Build history of the part. All positions in model axes, mm. Face numbers are marked on the shaded views. A direction names the side the tool comes from. Round coordinates to 2 decimals unless told otherwise and drop trailing zeros. Write each loop counter-clockwise with the first axis right and the second up, starting at its lowest first coordinate (ties: lowest second). Pieces come first, ordered by that corner, then holes.
from build123d import *

# Parameters (mm, degrees)
SKETCH_1_R          = 2.75
EXTRUDE_1_DEPTH     = 3
SKETCH_2_R          = 9
EXTRUDE_2_DEPTH     = 5.5
SKETCH_3_R          = 0.75
CUT_EXTRUDE_1_DEPTH = 7.5
CHAMFER_1_SIZE      = 0.7


with BuildPart() as part:
    # Эскиз1 → Бобышка-Вытянуть1 (new body)
    with BuildSketch(Plane.XY):
        Circle(SKETCH_1_R)
    extrude(amount=EXTRUDE_1_DEPTH)

    # Эскиз2 → Бобышка-Вытянуть2 (add)
    with BuildSketch(Plane.XY.offset(3)):
        Circle(SKETCH_2_R)
    extrude(amount=EXTRUDE_2_DEPTH)

    # Эскиз3 → Вырез-Вытянуть1 (cut)
    with BuildSketch(Plane.XY.offset(8.5)):
        Circle(SKETCH_3_R)
    extrude(amount=-CUT_EXTRUDE_1_DEPTH, mode=Mode.SUBTRACT)

    # Фаска1
    chamfer_1_edges = [part.edges().sort_by_distance(p)[0] for p in [
        (-0.75, 0, 1),
    ]]
    chamfer(chamfer_1_edges, length=CHAMFER_1_SIZE)


solid = part.part
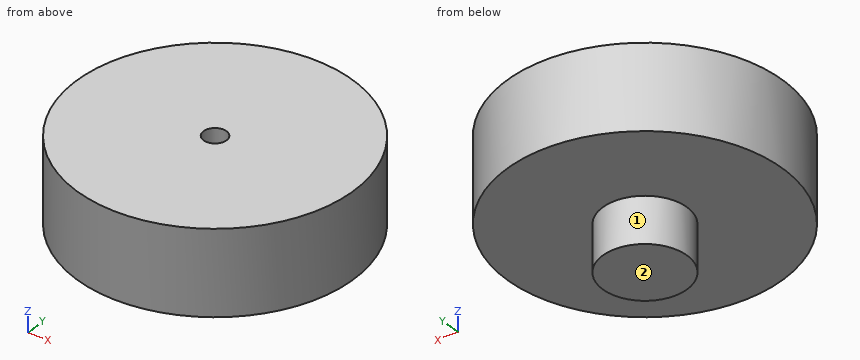
1) Which spindle directions (+Z, -Z, +X, -X, +Y, -Y) get a long thin tool onto all of the face, cutting with end or side? Do the marked faces 1 and 2. Say none if no direction does.
Results:
face 1: -Z
face 2: -Z, +X, -X, +Y, -Y
2) Slice it at B-B (x = -1). Write the cut outline in (y, z).
Results:
outline: (-8.94, 3) - (-2.56, 3) - (-2.56, 0) - (2.56, 0) - (2.56, 3) - (8.94, 3) - (8.94, 8.5) - (-8.94, 8.5) - close
3) Pin check, flat tips, straight feed: pin 1 Ø5 at (y, z) = (5.5, 2.5) entering from +X; pin 2 Ø1.5 at (y, z) = (4, 3.5) entering from -X; pin 3 Ø1.5 at (x, y) = (4.5, 1) entering from -Z. Stop position of each tip, or through.
Results:
pin 1: stops at x = 8.47
pin 2: stops at x = -8.39
pin 3: stops at z = 3
4) Slice it at A-A (z = 4.5). Write the cut outline in (x, y).
Results:
outline: circle Ø18 at (0, 0); hole circle Ø1.5 at (0, 0)
5) Slice it at C-C (z = 1.25). Write the cut outline in (x, y).
Results:
outline: circle Ø5.5 at (0, 0); hole circle Ø0.6 at (0, 0)
6) Wall check: L1, parallel to Y at x = 0, z = 5.5; L2, parallel to Z at x = -3, y = -5.5; L3, parallel to Y at x = 0.5, z = 6. Give the ranges that are in metal, low to high.
Results:
L1: y = -9 to -0.75, 0.75 to 9
L2: z = 3 to 8.5
L3: y = -8.99 to -0.56, 0.56 to 8.99
7) Slice it at D-D (x = 4.75). Write the cut outline in (y, z).
Results:
outline: (-7.64, 3) - (7.64, 3) - (7.64, 8.5) - (-7.64, 8.5) - close
